Read the model definition and answer for the solid it produces. Units are mm, in the model's axes. Face numbers are marked on the shaded views. Coordinates: 2 decimals unless noted, no trailing zeros. Order: outer loops, then holes, each group sorted by start corner. A loop starts at its lowest first (then second) coordinate and runs counter-clockwise, first axis right, second up. Notation, with made-up numbers: (-25.75, 88.5) - (13.25, 88.5) arc R17 ccw to (13.25, 108.5) - close; hole circle Ø4 at (2, -23.75). An arc over 180 degrees is marked (long way). Write item = value, one per line.
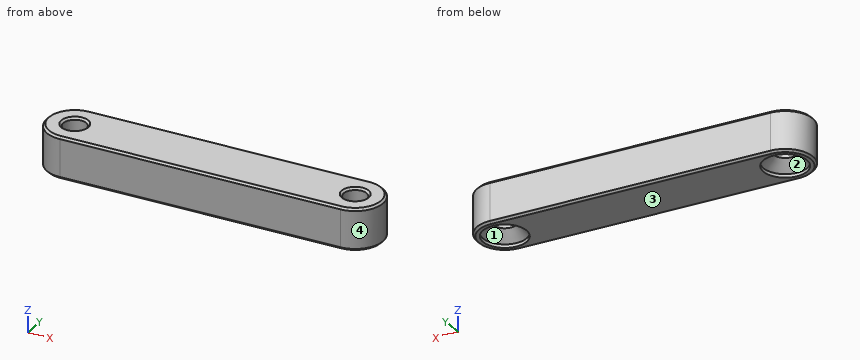
from build123d import *

# Parameters (mm, degrees)
SKETCH1_R                                    = 1.65
BOSS_EXTRUDE1_DEPTH                          = 6
CSK_FOR_M3_COUNTERSUNK_FLAT_HEAD_SCR_2_COUNT = 2
CSK_FOR_M3_COUNTERSUNK_FLAT_HEAD_SCR_2_PITCH = 40
CHAMFER1_SIZE                                = 0.3


with BuildPart() as part:
    # Sketch1 → Boss-Extrude1 (new body)
    with BuildSketch(Plane.XY):
        with BuildLine():
            Line((-20, 4), (20, 4))
            ThreePointArc((20, 4), (24, 0), (20, -4))
            Line((20, -4), (-20, -4))
            ThreePointArc((-20, -4), (-24, 0), (-20, 4))
        make_face()
        with Locations((-20, 0)):
            Circle(SKETCH1_R, mode=Mode.SUBTRACT)
        with Locations((20, 0)):
            Circle(SKETCH1_R, mode=Mode.SUBTRACT)
    extrude(amount=BOSS_EXTRUDE1_DEPTH)

    # Sketch3 → CSK for M3 Countersunk Flat Head Screw1 (revolve, cut)
    with BuildSketch(Plane.YZ.offset(-20)):
        Polygon((0, 0), (0, 6), (1.65, 6), (1.65, 2), (3.15, 0.5), (3.15, 0), align=None)
    csk_for_m3_countersunk_flat_head_screw1 = revolve(axis=Axis((-20, 0, -6.35), (0, 0, 1)), mode=Mode.SUBTRACT)

    # CSK for M3 Countersunk Flat Head Scr 2: CSK for M3 Countersunk Flat Head Screw1 ×2
    with Locations(*[(i * CSK_FOR_M3_COUNTERSUNK_FLAT_HEAD_SCR_2_PITCH, 0, 0) for i in range(1, CSK_FOR_M3_COUNTERSUNK_FLAT_HEAD_SCR_2_COUNT)]):
        add(csk_for_m3_countersunk_flat_head_screw1, mode=Mode.SUBTRACT)

    # Chamfer1
    chamfer1_edges = [part.edges().sort_by_distance(p)[0] for p in [
        (-21.65, 0, 6),
        (24, 0, 6),
        (18.35, 0, 6),
        (0, 4, 6),
        (-24, 0, 6),
        (0, 4, 0),
        (24, 0, 0),
        (0, -4, 0),
        (-24, 0, 0),
        (0, -4, 6),
    ]]
    chamfer(chamfer1_edges, length=CHAMFER1_SIZE)


solid = part.part
1) The part is cut by section A-A (z = 4.75). Determine the outline of the cut face in (x, y).
Returned:
outline = (-20, -4) - (20, -4) arc R4 ccw to (20, 4) - (-20, 4) arc R4 ccw to start; hole circle Ø3.3 at (-20, 0); hole circle Ø3.3 at (20, 0)
2) The part is cut by section C-C (y = 1.25). Count the separate pieces of the cut face and the enclosed holes in it, and give its area (3 significant figures).
Returned:
separate_pieces = 3
enclosed_holes = 0
area = 250 mm^2
3) A flat-ended cylindrical pin translates along its axis: pin 1 Ø3 at (y, z) = (-2, 2.5) entering from -X. Find the tip coordinate at first contact, or state that the pin passes through.
Returned:
pin_1 = -23.97
4) The part is cut by section B-B (z = 0.95). Determine the outline of the cut face in (x, y), and give its area (3 significant figures).
Returned:
outline = (-20, -4) - (20, -4) arc R4 ccw to (20, 4) - (-20, 4) arc R4 ccw to start; hole circle Ø5.4 at (-20, 0); hole circle Ø5.4 at (20, 0)
area = 324 mm^2
5) Determine the mould class of the marked faces 1, 2, 3 and 4 for opening direction X: pulls with the +X half, pulls with the -X half, needs draft (parallel to the pull), parting line crosses it, or undercut.
Returned:
face_1 = undercut
face_2 = undercut
face_3 = needs draft
face_4 = pulls with the +X half
6) Straight lines are drawn through the part: line 1 along X through (y, z) = (0, 3.1); line 2 along X through (y, z) = (0, 0.4); line 3 along Y through (x, z) = (20, 0.35). For each, find the intervals that lie inside material, in ascending order. Write a range as from..to.
Returned:
line_1 = -24..-21.65, -18.35..18.35, 21.65..24
line_2 = -24..-23.15, -16.85..16.85, 23.15..24
line_3 = -4..-3.15, 3.15..4
